Could you check a few things on this model? Use its own coordinates, in mm. A direction names the side the tool comes from. Coordinates: 2 decimals unless noted, no trailing zeros. Order: outer loops, then holes, each group sorted by start corner. A loop starts at its lowest first (then second) coordinate and runs counter-clockwise, first axis right, second up.
```python
from build123d import *

# Parameters (mm, degrees)
SKETCH1_W               = 70
SKETCH1_H               = 20
BOSS_EXTRUDE1_DEPTH     = 20
SKETCH2_W               = 10
SKETCH2_H               = 20
CUT_EXTRUDE1_DEPTH      = 20
SKETCH3_R               = 5
CUT_EXTRUDE2_DEPTH      = 60
SKETCH4_W               = 10
SKETCH4_H               = 20
CUT_EXTRUDE3_DEPTH      = 5
MIRROR3_COPY_1_SKETCH_W = 10
MIRROR3_COPY_1_SKETCH_H = 20
MIRROR3_COPY_1_DEPTH    = 5
SKETCH7_R               = 1.25
BOSS_EXTRUDE2_DEPTH     = 10


with BuildPart() as part:
    # Sketch1 → Boss-Extrude1 (new body)
    with BuildSketch(Plane.XY):
        Rectangle(SKETCH1_W, SKETCH1_H)
    extrude(amount=BOSS_EXTRUDE1_DEPTH)

    # Sketch2 → Cut-Extrude1 (cut)
    with BuildSketch(Plane.ZY.offset(35)):
        with Locations((10, 0)):
            Rectangle(SKETCH2_W, SKETCH2_H)
    cut_extrude1 = extrude(amount=-CUT_EXTRUDE1_DEPTH, mode=Mode.SUBTRACT)

    # Sketch3 → Cut-Extrude2 (cut)
    with BuildSketch(Plane.XY.offset(20)):
        with Locations((-25, 0)):
            Circle(SKETCH3_R)
    cut_extrude2 = extrude(amount=-CUT_EXTRUDE2_DEPTH, mode=Mode.SUBTRACT)

    # Sketch4 → Cut-Extrude3 (cut)
    with BuildSketch(Plane.XY.offset(20)):
        with Locations((-5, 0)):
            Rectangle(SKETCH4_W, SKETCH4_H)
    cut_extrude3 = extrude(amount=-CUT_EXTRUDE3_DEPTH, mode=Mode.SUBTRACT)

    # Mirror2: Cut-Extrude3 across plane
    add(cut_extrude3.mirror(Plane.XY.offset(10)), mode=Mode.SUBTRACT)

    # Mirror3: Cut-Extrude1, Cut-Extrude2, Cut-Extrude3 across plane
    add(cut_extrude1.mirror(Plane(origin=(0, 0, 0), x_dir=(0, 0, 1), z_dir=(1, 0, 0))), mode=Mode.SUBTRACT)
    add(cut_extrude2.mirror(Plane(origin=(0, 0, 0), x_dir=(0, 0, 1), z_dir=(1, 0, 0))), mode=Mode.SUBTRACT)
    add(cut_extrude3.mirror(Plane(origin=(0, 0, 0), x_dir=(0, 0, 1), z_dir=(1, 0, 0))), mode=Mode.SUBTRACT)

    # Mirror3 copy 1 sketch → Mirror3 copy 1 (cut)
    with BuildSketch(Plane(origin=(0, 0, 0), x_dir=(-1, 0, 0), z_dir=(0, 0, -1))):
        with Locations((-5, 0)):
            Rectangle(MIRROR3_COPY_1_SKETCH_W, MIRROR3_COPY_1_SKETCH_H)
    extrude(amount=-MIRROR3_COPY_1_DEPTH, mode=Mode.SUBTRACT)

    # Sketch7 → Boss-Extrude2 (add)
    with BuildSketch(Plane.XY.offset(15)):
        with BuildLine():
            Line((-10, -10), (-10, 15))
            ThreePointArc((-10, 15), (-7.5, 17.5), (-5, 15))
            Line((-5, 15), (-5, -10))
            Line((-5, -10), (-10, -10))
        make_face()
        with Locations((-7.5, 15)):
            Circle(SKETCH7_R, mode=Mode.SUBTRACT)
    boss_extrude2 = extrude(amount=BOSS_EXTRUDE2_DEPTH)

    # Mirror4: Boss-Extrude2 across plane
    add(boss_extrude2.mirror(Plane.XY.offset(10)))


solid = part.part
```
Item 1: I need wall thicknesses on line 1 (Z direction, x = 26, y = -8.5); line 2 (X direction, y = 8, z = 2.5); line 3 (Y direction, x = -25, z = 2.7). Which ranges of each line are inside material? Lowest first, please.
Item 2: For pin 1 Ø5 at (x, z) = (21, 13) entering from -Y; pin 2 Ø16 at (x, y) = (23, -1.5) entering from +Z; pin 3 Ø1.5 at (y, z) = (0.5, 11) entering from -X; pin 4 Ø1.5 at (x, z) = (-1.5, 10) entering from +Y, each with a flat end and sliding along its axis, tell me the tip position at first contact or that it passes through.
Item 3: Suppose I cut it at D-D (z = -1.25). List the corners of the cut face in (x, y) for me, and give its area (3 significant figures).
Item 4: Thinking about a two-plate mould opening in Z: for faces 1 (the face through (-27, -5, 5)), 2 (the face through (19.5, 0.1, 20)), 3 (the face through (30, 0, 18)), which applies, +Z half, -Z half, draft (parallel to the pull), parting line (faces both ways), or undercut?
Item 5: Which directions (+Z, -Z, +X, -X, +Y, -Y) give clear straight access to the entire face, cutting with the end or side of a thin tool? Please do faces 4 (the face through (19.5, 0.1, 0)), 5 (the face through (-7, 13, 15)), 6 (the face through (27, -5, 15)).
Item 6: Suppose I cut it at C-C (x = -7.5). List the corners of the cut face in (y, z) for me.
Item 7: Suppose I cut it at B-B (x = 25). List the corners of the cut face in (y, z) for me.
Item 8: Suppose I cut it at A-A (z = 4). List the corners of the cut face in (x, y) for me, and give its area (3 significant figures).
Geometry results:
1. line 1: z = 0 to 5, 15 to 20
1. line 2: x = -35 to -5, 10 to 35
1. line 3: y = -10 to -5, 5 to 10
2. pin 1: stops at y = -10
2. pin 2: stops at z = 20
2. pin 3: stops at x = -15
2. pin 4: stops at y = 10
3. outline: (-10, -10) - (-5, -10) - (-5, 15) arc R2.5 ccw to (-10, 15) - close; hole circle Ø2.5 at (-7.5, 15)
3. area: 130 mm2
4. face 1: undercut
4. face 2: +Z half
4. face 3: draft
5. face 4: -Z, +X, +Y, -Y
5. face 5: +X, -X, +Y
5. face 6: +X, +Y, -Y
6. outline: (-10, -5) - (13.75, -5) - (13.75, 5) - (10, 5) - (10, 15) - (13.75, 15) - (13.75, 25) - (-10, 25) - close; (16.25, -5) - (17.5, -5) - (17.5, 5) - (16.25, 5) - close; (16.25, 15) - (17.5, 15) - (17.5, 25) - (16.25, 25) - close
7. outline: (-10, 0) - (-5, 0) - (-5, 5) - (-10, 5) - close; (-10, 15) - (-5, 15) - (-5, 20) - (-10, 20) - close; (5, 0) - (10, 0) - (10, 5) - (5, 5) - close; (5, 15) - (10, 15) - (10, 20) - (5, 20) - close
8. outline: (-35, -10) - (-5, -10) - (-5, 15) arc R2.5 ccw to (-10, 15) - (-10, 10) - (-35, 10) - close; (10, -10) - (35, -10) - (35, 10) - (10, 10) - close; hole circle Ø10 at (-25, 0); hole circle Ø2.5 at (-7.5, 15); hole circle Ø10 at (25, 0)
8. area: 973 mm2
